Geometry check sheet. Reference: the model listing, model coordinates, mm. A direction names the side the tool comes from. Round coordinates to 2 decimals unless told otherwise and drop trailing zeros. Write each loop counter-clockwise with the first axis right and the second up, starting at its lowest first coordinate (ties: lowest second). Pieces come first, ordered by that corner, then holes. Notation, with made-up numbers: M -30,19 L -17,19 A7 cw -17,31 Z; hole C -29.5,60.5 d4. An arc over 180 degrees is marked long. One line per item, written item: value. Start each with the question number.
1. Scan lines: probe 1 along Z at (x, y) = (-100, 14.55); probe 2 along Z at (x, y) = (70, 8.75); probe 3 along Z at (x, y) = (-59.5, 1). Record each from-to range of solid material in increasing order. Write a range as [from, to].
2. Depth check by flat-ended pin: P1, Ø3, axis at y = 9.5, z = -44, coming from the +X side; P2, Ø6, axis at x = -97.5, z = 73, coming from the +Y side; P3, Ø0.8, axis at y = 8, z = 94, coming from the +X side; P4, Ø11, axis at x = -100, z = -70, coming from the +Y side. Enter the tip coordinate at first touch or a pass-through.
3. Section check A-A (z = -70). Record the boundary of the cut face in (x, y), and give its area (3 significant figures).
4. Section check C-C (x = 100). Record the boundary of the cut face in (y, z).
5. Release check for a two-part mould opening along Z. For faces 1 (the flat face through (124.5, 15, 1)), 2 (the flat face through (-120.75, 8, -1)), 3 (the cylindrical face through (121.995, 8.381, 95.877)), 4 (the flat face through (-100, 13.5, -70)) record: pulls with the +Z half, pulls with the -Z half, needs draft (parallel to the pull), parting line crosses it, or undercut.
6. Access from +Z, -Z, +X, -X, +Y, -Y to the whole of each face (thin tool, end or side, straight path). Record for faces 5 (the flat face through (114, 8, 94)), 6 (the cylindrical face through (104.42, 15.27, 74.06)), 7 (the cylindrical face through (-122.696, 8.381, 95.289)).
7. Section check B-B (y = 8.5). Record the boundary of the cut face in (x, z), and give its area (3 significant figures).
8. Section check D-D (z = 33.5). Record the boundary of the cut face in (x, y).
Autodesk Fusion 360 part; units mm, degrees
sketch "Sketch1" plane through (0, 0, 0) normal (0, 1, 0) x (1, 0, 0)
  line L0 (118.5, 97) -> (-118.5, 97)
  line L1 (-124.5, 91) -> (-124.5, -91)
  line L2 (-118.5, -97) -> (118.5, -97)
  line L3 (124.5, -91) -> (124.5, 91)
  line L4 (124.5, 97) -> (-124.5, -97) construction
  line L5 (-124.5, 97) -> (124.5, -97) construction
  arc A0 (118.5, -97) -> (124.5, -91) centre (118.5, -91) ccw
  arc A1 (-124.5, -91) -> (-118.5, -97) centre (-118.5, -91) ccw
  arc A2 (124.5, 91) -> (118.5, 97) centre (118.5, 91) ccw
  arc A3 (-118.5, 97) -> (-124.5, 91) centre (-118.5, 91) ccw
  dimension "d1" = 249
  dimension "d2" = 194
  dimension "d3" = 6
  dimension "d4" = 6
  dimension "d5" = 6
  dimension "d6" = 6
extrude "Extrude1" add sketch "Sketch1" along normal blind 17
sketch "Sketch2" plane through (0, 0, 0) normal (0, 1, 0) x (1, 0, 0)
  line L0 (115.75, 93.25) -> (-115.75, 93.25)
  line L1 (-120.75, 88.25) -> (-120.75, -88.25)
  line L2 (-115.75, -93.25) -> (115.75, -93.25)
  line L3 (120.75, -88.25) -> (120.75, 88.25)
  line L4 (120.75, 93.25) -> (-120.75, -93.25) construction
  line L5 (-120.75, 93.25) -> (120.75, -93.25) construction
  arc A0 (-120.75, -88.25) -> (-115.75, -93.25) centre (-115.75, -88.25) ccw
  arc A1 (115.75, -93.25) -> (120.75, -88.25) centre (115.75, -88.25) ccw
  arc A2 (-115.75, 93.25) -> (-120.75, 88.25) centre (-115.75, 88.25) ccw
  arc A3 (120.75, 88.25) -> (115.75, 93.25) centre (115.75, 88.25) ccw
  dimension "d9" = 241.5
  dimension "d10" = 186.5
  dimension "d11" = 5
  dimension "d12" = 5
  dimension "d13" = 5
  dimension "d14" = 5
ref_plane "WorkPlane1" through (0, 3, 0) normal (0, 1, 0) x (-1, 0, 0)
extrude "Extrude2" cut sketch "Sketch2" along normal blind 9.3
sketch "Sketch3" plane through (0, 0, 0) normal (0, -1, 0) x (1, 0, 0)
  line L0 (120.75, 88.25) -> (120.75, -88.25)
  arc A0 (115.75, -93.25) -> (120.75, -88.25) centre (115.75, -88.25) ccw
  line L1 (115.75, -93.25) -> (-115.75, -93.25)
  arc A1 (-120.75, -88.25) -> (-115.75, -93.25) centre (-115.75, -88.25) ccw
  line L2 (-120.75, -88.25) -> (-120.75, 88.25)
  arc A2 (-115.75, 93.25) -> (-120.75, 88.25) centre (-115.75, 88.25) ccw
  line L3 (-115.75, 93.25) -> (115.75, 93.25)
  arc A3 (120.75, 88.25) -> (115.75, 93.25) centre (115.75, 88.25) ccw
  arc A4 (-124.5, -91) -> (-118.5, -97) centre (-118.5, -91) ccw
  line L4 (-118.5, -97) -> (118.5, -97)
  arc A5 (118.5, -97) -> (124.5, -91) centre (118.5, -91) ccw
  line L5 (124.5, -91) -> (124.5, 91)
  arc A6 (124.5, 91) -> (118.5, 97) centre (118.5, 91) ccw
  line L6 (118.5, 97) -> (-118.5, 97)
  arc A7 (-118.5, 97) -> (-124.5, 91) centre (-118.5, 91) ccw
  line L7 (-124.5, 91) -> (-124.5, -91)
  line L8 (-113.5, 89) -> (113.5, 89)
  line L9 (116.5, 86) -> (116.5, -89)
  line L10 (116.5, -89) -> (-113.5, -89)
  line L11 (-116.5, -86) -> (-116.5, 86)
  line L12 (-116.5, 89) -> (116.5, -89) construction
  line L13 (116.5, 89) -> (-116.5, -89) construction
  arc A8 (-113.5, 89) -> (-116.5, 86) centre (-113.5, 86) ccw
  arc A9 (116.5, 86) -> (113.5, 89) centre (113.5, 86) ccw
  arc A10 (-116.5, -86) -> (-113.5, -89) centre (-113.5, -86) ccw
  dimension "d18" = 233
  dimension "d19" = 178
  dimension "d20" = 3
  dimension "d21" = 3
  dimension "d22" = 3
sketch "Sketch4" plane through (124.5, 0, 0) normal (1, 0, 0) x (0, 1, 0)
  line L0 (0, 91) -> (0, -91)
  line L1 (0, -91) -> (17, -91)
  line L2 (17, -91) -> (17, 91)
  line L3 (17, 91) -> (0, 91)
  line L4 (3, 94) -> (12.2, 94)
  line L5 (12.2, 94) -> (12.2, -94)
  line L6 (12.2, -94) -> (3, -94)
  line L7 (3, -94) -> (3, 94)
  dimension "d23" = 9.2
  dimension "d24" = 188
extrude "Extrude3" cut sketch "Sketch4" against normal blind 6 contours L3 L4 L5 L7 | L1 L3 L5 L7 | L1 L5 L6 L7
sketch "Sketch5" plane through (0, 17, 0) normal (0, 1, 0) x (-1, 0, 0)
  arc A0 (118.5, -97) -> (124.5, -91) centre (118.5, -91) ccw
  line L0 (124.5, -91) -> (124.5, 91)
  arc A1 (124.5, 91) -> (118.5, 97) centre (118.5, 91) ccw
  line L1 (118.5, 97) -> (-118.5, 97)
  arc A2 (-118.5, 97) -> (-124.5, 91) centre (-118.5, 91) ccw
  line L2 (-124.5, 91) -> (-124.5, -91)
  arc A3 (-124.5, -91) -> (-118.5, -97) centre (-118.5, -91) ccw
  line L3 (-118.5, -97) -> (118.5, -97)
  circle A4 centre (-100, 70) radius 6
  circle A5 centre (100, 70) radius 6
  circle A6 centre (-100, -70) radius 6
  circle A7 centre (100, -70) radius 6
  dimension "d27" = 12
  dimension "d28" = 12
  dimension "d29" = 12
  dimension "d30" = 12
extrude "Extrude4" cut sketch "Sketch5" against normal blind 3.5 contours A4 | A5 | A6 | A7
extrude "Extrude5" add sketch "Sketch3" against normal blind 3 contours L0 A0 L1 A1 L2 A2 L3 A3
sketch "Sketch6" plane through (118.5, 0, 0) normal (1, 0, 0) x (0, 1, 0)
  line L0 (9.3, -92.4258) -> (3, -92.4258)
  line L1 (3, -92.4258) -> (3, -94)
  line L2 (3, -94) -> (12.2, -94)
  line L3 (12.2, -94) -> (12.2, 94)
  line L4 (12.2, 94) -> (3, 94)
  line L5 (3, 94) -> (3, 92.4258)
  line L6 (3, 92.4258) -> (9.3, 92.4258)
  line L7 (9.3, 92.4258) -> (9.3, -92.4258)
  line L8 (3, 94) -> (12.2, 94)
  line L9 (12.2, 94) -> (12.2, -94)
  line L10 (12.2, -94) -> (3, -94)
  line L11 (3, -94) -> (3, 94)
extrude "Extrude6" cut sketch "Sketch6" against normal blind 15
sketch "Sketch7" plane through (0, 3, 0) normal (0, 1, 0) x (1, 0, 0)
extrude "Extrude7" cut 1 faces at (-42.6667, 9.3, -31.0833) along direction (0, 1, 0) blind 3
Result sheet:
1. probe 1: z = [-97, -76], [-64, 64], [76, 97]
1. probe 2: z = [-97, -93.25], [93.25, 97]
1. probe 3: z = [-97, -89], [89, 97]
2. P1: stops at x = -120.75
2. P2: stops at y = 17
2. P3: stops at x = 123.7
2. P4: stops at y = 13.5
3. outline: M -124.5,0 L -116.5,0 L -116.5,3 L -120.75,3 L -120.75,12.3 L 103.5,12.3 L 103.5,12.2 L 124.5,12.2 L 124.5,17 L 106,17 L 106,13.5 L 94,13.5 L 94,17 L -94,17 L -94,13.5 L -106,13.5 L -106,17 L -124.5,17 Z; M 116.5,0 L 124.5,0 L 124.5,3 L 116.5,3 Z
3. area: 1,170 mm2
4. outline: M 0,-97 L 17,-97 L 17,-76 L 13.5,-76 L 13.5,-64 L 17,-64 L 17,64 L 13.5,64 L 13.5,76 L 17,76 L 17,97 L 0,97 L 0,89 L 3,89 L 3,93.25 L 12.3,93.25 L 12.3,-93.25 L 3,-93.25 L 3,-89 L 0,-89 Z
5. face 1: needs draft
5. face 2: undercut
5. face 3: pulls with the +Z half
5. face 4: undercut
6. face 5: +X
6. face 6: +Y
6. face 7: +Z, -X, +Y, -Y
7. outline: M -124.5,-91 A6 ccw -118.5,-97 L 118.5,-97 A6 ccw 123.7,-94 L 103.5,-94 L 103.5,-93.25 L -115.75,-93.25 A5 cw -120.75,-88.25 L -120.75,88.25 A5 cw -115.75,93.25 L 103.5,93.25 L 103.5,94 L 123.7,94 A6 ccw 118.5,97 L -118.5,97 A6 ccw -124.5,91 Z
7. area: 2,520 mm2
8. outline: M -124.5,0 L -116.5,0 L -116.5,3 L -120.75,3 L -120.75,12.3 L 103.5,12.3 L 103.5,12.2 L 124.5,12.2 L 124.5,17 L -124.5,17 Z; M 116.5,0 L 124.5,0 L 124.5,3 L 116.5,3 Z
